```python
from build123d import *

# Parameters (mm, degrees)
SKETCH1_W           = 600
SKETCH1_H           = 600
BOSS_EXTRUDE1_DEPTH = 1200
SHELL1_T            = -25
SKETCH2_R           = 6
BOSS_EXTRUDE2_DEPTH = 5


with BuildPart() as part:
    # Sketch1 → Boss-Extrude1 (new body)
    with BuildSketch(Plane(origin=(0, 0, 0), x_dir=(0, 0, -1), z_dir=(1, 0, 0))):
        with Locations((300, 300)):
            Rectangle(SKETCH1_W, SKETCH1_H)
    extrude(amount=BOSS_EXTRUDE1_DEPTH)

    # Shell1
    shell1_openings = [part.faces().sort_by_distance(p)[0] for p in [
        (1200, 300, -300),
    ]]
    offset(amount=SHELL1_T, openings=shell1_openings, kind=Kind.INTERSECTION)

    # Sketch2 → Boss-Extrude2 (add)
    with BuildSketch(Plane.XY):
        with Locations(Location((1050, 80, 0), (0, 0, 180))):
            Circle(SKETCH2_R)
    boss_extrude2 = extrude(amount=BOSS_EXTRUDE2_DEPTH)

    # Mirror1: Boss-Extrude2 across plane
    add(boss_extrude2.mirror(Plane.XY.offset(-300)))


solid = part.part
```
Source: CAD feature listing. Evaluate the final solid. Frame: model axes, mm. A direction names the side the tool comes from. Give positions to 0.01 mm unless a question says otherwise; leave off trailing zeros. Order: outer loops, then holes, each group sorted by start corner. A loop starts at its lowest first (then second) coordinate and runs counter-clockwise, first axis right, second up.
(1) Section query C-C (z = -461.5). Return the cut outline in (x, y), plus the area to 4 significant figures.
(2) Contact query for flat-ended pins moving along their axis: P1, Ø1.5, axis at x = 452.5, y = 98, coming from the +Z side; P2, Ø5, axis at x = 946, y = 318.5, coming from the -Z side. Output: stop coordinate, or through.
(3) Section query A-A (x = 897). Return the cut outline in (y, z).
(4) Access query for faces 1 (the face through (1200, 13, -276)), 2 (the face through (604, 575, -296)). Directions: +Z, -Z, +X, -X, +Y, -Y. A direction counts if a zero-diameter tool reaches every point of the face in a straight line with its end or side. Return the directions, or none.
(5) Material intervals for line 1 along Y through (x, z) = (726.5, -78.5); line 2 along Z through (x, y) = (262, 78); line 3 along X through (y, z) = (496.5, -131), sorted ascending.
(6) Pull-direction query (Y, two-part tool) for faces 3 (the face through (604, 296, -575)), 4 (the face through (592, 600, -296)), 5 (the face through (592, 296, 0)); classes: +Y half, -Y half, draft (parallel to the pull), parting line (faces both ways), or undercut.
(7) Section query B-B (y = 123). Return the cut outline in (x, z).
Outcome:
1. outline: (0, 0) - (1200, 0) - (1200, 25) - (25, 25) - (25, 575) - (1200, 575) - (1200, 600) - (0, 600) - close
1. area: 73,750 mm2
2. P1: stops at z = 0
2. P2: stops at z = -600
3. outline: (0, -600) - (600, -600) - (600, 0) - (0, 0) - close; hole (25, -575) - (575, -575) - (575, -25) - (25, -25) - close
4. face 1: +Z, -Z, +X, +Y, -Y
4. face 2: +X
5. line 1: y = 0 to 25, 575 to 600
5. line 2: z = -600 to -575, -25 to 0
5. line 3: x = 0 to 25
6. face 3: undercut
6. face 4: +Y half
6. face 5: draft
7. outline: (0, -600) - (1200, -600) - (1200, -575) - (25, -575) - (25, -25) - (1200, -25) - (1200, 0) - (0, 0) - close
